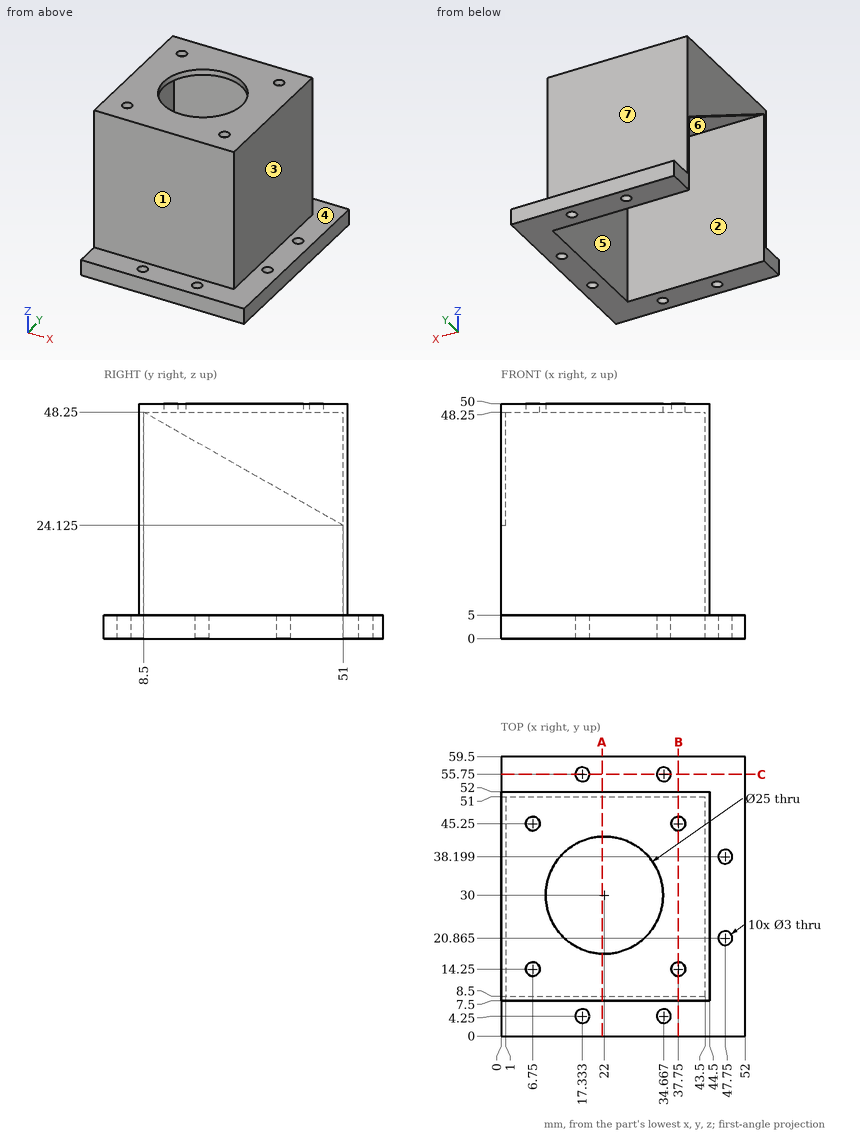
Could you check a few things on this drawing? It's one solid part, dimensions in mm from its lowest x, y, z. A direction names the side the tool comes from. Round coordinates to 2 decimals unless told otherwise and drop trailing zeros. Order: outer loops, then holes, each group sorted by start corner. A loop starts at its lowest first (then second) coordinate and runs counter-clockwise, first axis right, second up. Notation, with made-up numbers: M -1.5,79.25 L 39.5,79.25 A24 cw 39.5,113.25 Z; hole C 71,58 d7. An arc over 180 degrees is marked long. Use a Markdown table: item, result.
1) I'm going to push flat-ended pins straight in: P1, Ø21, axis at x = 12.5, y = 20.5, coming from the -Z side; P2, Ø3, axis at y = 45.5, z = 19, coming from the -X side; P3, Ø1, axis at x = 10.5, z = 16.5, coming from the -Y side; P4, Ø3.5, axis at x = 47.75, y = 38.2, coming from the -Z side. Where does each tip first touch, or does it pass through?
Geometry says:
| item | result |
|---|---|
| P1 | stops at z = 48.25 |
| P2 | stops at x = 43.5 |
| P3 | stops at y = 7.5 |
| P4 | stops at z = 0 |
2) If I drill on line 1 along X through (y, z) = (45.25, 49.5); line 2 along Y through (x, z) = (37, 36); line 3 along X through (y, z) = (27.5, 40.5), over which ranges is the centre line in solid material (lowest first)?
Geometry says:
| item | result |
|---|---|
| line 1 | x = 0 to 5.25, 8.25 to 36.25, 39.25 to 44.5 |
| line 2 | y = 7.5 to 8.5, 51 to 52 |
| line 3 | x = 0 to 1, 43.5 to 44.5 |
3) Imagine slicing it at B-B (x = 37.75). List the corners of the cut face in (y, z) for me, then the cut area to 3 significant figures.
Geometry says:
| item | result |
|---|---|
| outline | M 0,0 L 8.5,0 L 8.5,48.25 L 12.75,48.25 L 12.75,50 L 7.5,50 L 7.5,5 L 0,5 Z; M 15.75,48.25 L 43.75,48.25 L 43.75,50 L 15.75,50 Z; M 46.75,48.25 L 51,48.25 L 51,0 L 59.5,0 L 59.5,5 L 52,5 L 52,50 L 46.75,50 Z |
| area | 239 mm² |
4) Imagine slicing it at A-A (x = 21.5). List the corners of the cut face in (y, z) for me.
Geometry says:
| item | result |
|---|---|
| outline | M 0,0 L 8.5,0 L 8.5,48.25 L 17.51,48.25 L 17.51,50 L 7.5,50 L 7.5,5 L 0,5 Z; M 42.49,48.25 L 51,48.25 L 51,0 L 59.5,0 L 59.5,5 L 52,5 L 52,50 L 42.49,50 Z |
5) Imagine slicing it at C-C (y = 55.75). List the corners of the cut face in (x, z) for me.
Geometry says:
| item | result |
|---|---|
| outline | M 0,0 L 15.83,0 L 15.83,5 L 0,5 Z; M 18.83,0 L 33.17,0 L 33.17,5 L 18.83,5 Z; M 36.17,0 L 52,0 L 52,5 L 36.17,5 Z |
6) On a 3-axis mill with a long thin cutter (end or side, diameter ignored), from which of +Z, -Z, +X, -X, +Y, -Y can I reach the whole of each face in a straight line? I mean the marked faces 1, 2 and 3. Say none if no direction works.
Geometry says:
| item | result |
|---|---|
| face 1 | +Z, +X, -X, -Y |
| face 2 | -Z, -X |
| face 3 | +Z, +X, +Y, -Y |
7) If we mould it in two halves opening along Y, with no side actions, what happens to the marked faces 4, 5, 6 and 7? For each: +Y half, -Y half, draft (parallel to the pull), parting line (faces both ways), or undercut.
Geometry says:
| item | result |
|---|---|
| face 4 | draft |
| face 5 | undercut |
| face 6 | undercut |
| face 7 | +Y half |
